Geometry check sheet. Reference: the model listing, model coordinates, mm. Give positions to 0.01 mm unless a question says otherwise; leave off trailing zeros. Write each loop counter-clockwise with the first axis right and the second up, starting at its lowest first coordinate (ties: lowest second). Pieces come first, ordered by that corner, then holes. Notation, with made-up numbers: M 35,69 L 75,69 A27 ccw 75,99 Z; hole C 40,84.25 d5. An arc over 180 degrees is marked long. One line per item, written item: value. Start each with the question number.
1. Cross-section at A-A on x = 0. Record the cut outline in (y, z).
2. Scan lines: line 1 (X direction, y = 1.3, z = 0); line 2 (Z direction, x = 5, y = 0.4); line 3 (X direction, y = 1.2, z = 5.5). Record each from-to range of solid material in increasing order.
3. Cross-section at B-B on y = 0.95. Record the cut outline in (x, z), then the cut area to 3 significant figures.
4. Cross-section at C-C on z = -33. Record the cut outline in (x, y).
5. Cross-section at D-D on x = -33. Record the cut outline in (y, z).
from build123d import *

# Parameters (mm, degrees)
SKETCH1_R           = 6
SKETCH1_R_2         = 3
BOSS_EXTRUDE1_DEPTH = 3


with BuildPart() as part:
    # Sketch1 → Boss-Extrude1 (new body)
    with BuildSketch(Plane(origin=(0, 0, 0), x_dir=(1, 0, 0), z_dir=(0, 1, 0))):
        with BuildLine():
            Line((24, -39.5), (34.5, -39.5))
            ThreePointArc((34.5, -39.5), (38.035533906, -38.035533906), (39.5, -34.5))
            Line((39.5, -34.5), (39.5, -24))
            Line((39.5, -24), (39.5, 24))
            Line((39.5, 24), (65.757128891, 24))
            ThreePointArc((65.757128891, 24), (-49.497474683, 49.497474683), (-24, -65.757128891))
            Line((-24, -65.757128891), (-24, -39.5))
            Line((-24, -39.5), (24, -39.5))
        make_face()
        with Locations(Location((0, 0, 0), (0, 0, 270))):
            Circle(SKETCH1_R, mode=Mode.SUBTRACT)
        with Locations(Location((33, 0, 0), (0, 0, 270))):
            Circle(SKETCH1_R_2, mode=Mode.SUBTRACT)
        with Locations(Location((0, -33, 0), (0, 0, 270))):
            Circle(SKETCH1_R_2, mode=Mode.SUBTRACT)
        with Locations(Location((-33, 0, 0), (0, 0, 270))):
            Circle(SKETCH1_R_2, mode=Mode.SUBTRACT)
        with Locations(Location((0, 33, 0), (0, 0, 270))):
            Circle(SKETCH1_R_2, mode=Mode.SUBTRACT)
    extrude(amount=BOSS_EXTRUDE1_DEPTH)


solid = part.part
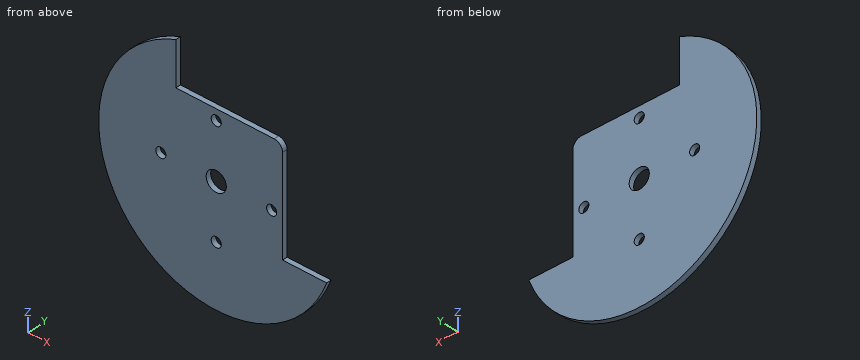
Report:
1. outline: M 0,-70 L 3,-70 L 3,-36 L 0,-36 Z; M 0,-30 L 3,-30 L 3,-6 L 0,-6 Z; M 0,6 L 3,6 L 3,30 L 0,30 Z; M 0,36 L 3,36 L 3,39.5 L 0,39.5 Z
2. line 1: x = -70 to -36, -30 to -6, 6 to 30, 36 to 39.5
2. line 2: z = -69.82 to -3.32, 3.32 to 39.5
2. line 3: x = -69.78 to -2.4, 2.4 to 39.5
3. outline: M -24,39.5 L -24,65.76 A70 ccw long 65.76,-24 L 39.5,-24 L 39.5,34.5 A5 ccw 34.5,39.5 Z; hole C -33,0 d6; hole C 0,0 d12; hole C 0,-33 d6; hole C 0,33 d6; hole C 33,0 d6
3. area: 11,500 mm^2
4. outline: M -61.73,0 L -3,0 L -3,3 L -61.73,3 Z; M 3,0 L 61.73,0 L 61.73,3 L 3,3 Z
5. outline: M 0,-61.73 L 3,-61.73 L 3,-3 L 0,-3 Z; M 0,3 L 3,3 L 3,61.73 L 0,61.73 Z
